from build123d import *

# Parameters (mm, degrees)
SKETCH_3_R      = 1.35
SKETCH_3_R_2    = 1
EXTRUDE_2_DEPTH = 3


with BuildPart() as part:
    # 草图3 → 凸台-拉伸2 (new body)
    with BuildSketch(Plane.XY):
        with BuildLine():
            Line((21.499968123, 3.52141019), (16.156278552, 3.52141019))
            add(Edge.make_bspline(
                [(16.156278552, 3.52141019), (16.088160339, 5.051537173), (14.821900334, 5.873909505)],
                knots=[0, 0, 0, 1, 1, 1], degree=2))
            Line((14.821900334, 5.873909505), (8.771282217, 5.873909505))
            add(Edge.make_bspline(
                [(7.754778373, 3.595279655), (7.816403966, 4.944689103), (8.771282217, 5.873909505)],
                knots=[0, 0, 0, 1, 1, 1], degree=2))
            Line((7.754778373, 3.595279655), (1.868346732, 3.595279655))
            ThreePointArc((1.868346732, 3.595279655), (-3.997767344, 0.192060873), (1.627998751, -3.595279655))
            Line((1.627998751, -3.595279655), (7.754778373, -3.595279655))
            add(Edge.make_bspline(
                [(7.754778373, -3.595279655), (7.816403966, -4.944689103), (8.771282217, -5.873909505)],
                knots=[0, 0, 0, 1, 1, 1], degree=2))
            Line((8.771282217, -5.873909505), (14.821900334, -5.873909505))
            add(Edge.make_bspline(
                [(16.156278552, -3.52141019), (16.088160339, -5.051537173), (14.821900334, -5.873909505)],
                knots=[0, 0, 0, 1, 1, 1], degree=2))
            Line((16.156278552, -3.52141019), (21.499968123, -3.52141019))
            ThreePointArc((21.499968123, -3.52141019), (23.982399961, -2.488702667), (24.999902637, 0))
            ThreePointArc((24.999902637, 0), (23.982399961, 2.488702667), (21.499968123, 3.52141019))
        make_face()
        with Locations((0, 0.058433534)):
            Circle(SKETCH_3_R, mode=Mode.SUBTRACT)
        with Locations((10.35, 0)):
            Circle(SKETCH_3_R_2, mode=Mode.SUBTRACT)
        with Locations((14.31, 0)):
            Circle(SKETCH_3_R_2, mode=Mode.SUBTRACT)
        with Locations((21.499968123, 0.02141019)):
            Circle(SKETCH_3_R, mode=Mode.SUBTRACT)
    extrude(amount=EXTRUDE_2_DEPTH)


solid = part.part
Geometry: final body of the model. Coordinates: model frame, mm. A direction names the side the tool comes from. Coordinates: 2 decimals unless noted, no trailing zeros. Write each loop counter-clockwise with the first axis right and the second up, starting at its lowest first coordinate (ties: lowest second). Pieces come first, ordered by that corner, then holes. Notation, with made-up numbers: (-17, 78.25) - (33, 78.25) arc R14 ccw to (33, 103.25) - close; hole circle Ø11 at (80.5, 81). An arc over 180 degrees is marked (long way). Return JSON: item names as keys, results as strings.
Item 1: Pull-direction query (Y, two-part tool) for faces 1 (the face through (12, 5.874, 1)), 2 (the face through (10.3, 1.4, 0)), 3 (the face through (-1.071, -0.763, 1.479)); classes: +Y half, -Y half, draft (parallel to the pull), parting line (faces both ways), or undercut.
Completed:
{"face 1": "+Y half", "face 2": "draft", "face 3": "undercut"}
Item 2: Section query D-D (z = 2.5). Count the separate pieces of the cut face and the enclosed holes in it, and give its area (3 significant figures).
Completed:
{"separate pieces": "1", "enclosed holes": "4", "area": "216 mm2"}
Item 3: Section query A-A (x = 14.31). Output: boundary loops of the cut face in (y, z).
Completed:
{"outline": "(-5.87, 0) - (-1, 0) - (-1, 3) - (-5.87, 3) - close; (1, 0) - (5.87, 0) - (5.87, 3) - (1, 3) - close"}
Item 4: Pin query (flat end, axial travel): pin 1 Ø1.6 at (x, y) = (10.35, 0) entering from +Z; pin 2 Ø0.9 at (x, z) = (19, 1) entering from -Y; pin 3 Ø1.5 at (x, z) = (18, 2) entering from +Y; pin 4 Ø1 at (y, z) = (-1, 0.5) entering from +X. Return the tip coordinate at first contact, or that it passes through.
Completed:
{"pin 1": "passes through", "pin 2": "stops at y = -3.52", "pin 3": "stops at y = 3.52", "pin 4": "stops at x = 24.97"}
Item 5: Section query C-C (x = 0). Output: boundary loops of the cut face in (y, z).
Completed:
{"outline": "(-3.94, 0) - (-1.29, 0) - (-1.29, 3) - (-3.94, 3) - close; (1.41, 0) - (4.06, 0) - (4.06, 3) - (1.41, 3) - close"}
Item 6: Reachability of faces 4 (the face through (19, -3.521, 1)), 5 (the face through (19, 3.521, 1)), 6 (the face through (5, 3.595, 1)), 7 (the face through (5, -3.595, 1)) from +Z, -Z, +X, -X, +Y, -Y: full face, straight path, thin tool, end or side. Return the list, or none.
Completed:
{"face 4": "+Z, -Z, +X, -Y", "face 5": "+Z, -Z, +X, +Y", "face 6": "+Z, -Z, +Y", "face 7": "+Z, -Z, -Y"}
Item 7: Section query B-B (y = 0.5). Output: boundary loops of the cut face in (x, z), and give its area (3 significant figures).
Completed:
{"outline": "(-3.98, 0) - (-1.28, 0) - (-1.28, 3) - (-3.98, 3) - close; (1.28, 0) - (9.48, 0) - (9.48, 3) - (1.28, 3) - close; (11.22, 0) - (13.44, 0) - (13.44, 3) - (11.22, 3) - close; (15.18, 0) - (20.24, 0) - (20.24, 3) - (15.18, 3) - close; (22.76, 0) - (24.97, 0) - (24.97, 3) - (22.76, 3) - close", "area": "61.2 mm2"}
Item 8: Line query: L1, parallel to Y at x = 0, z = 0.65; L2, parallel to Y at x = 21.5, z = 2.75; L3, parallel to Y at x = 19.75, z = 1.9. Output: solid intervals per line, ascending.
Completed:
{"L1": "y = -3.94 to -1.29, 1.41 to 4.06", "L2": "y = -3.52 to -1.33, 1.37 to 3.52", "L3": "y = -3.52 to 3.52"}
